```python
from build123d import *

# Parameters (mm, degrees)
F3_DEPTH      = 1400
F4_R          = 12
F4_R_2        = 8
F5_DEPTH      = 3
F5_DEPTH_BACK = 43
F6_DEPTH      = 63
F4_R_3        = 2
F7_DEPTH      = 50000


with BuildPart() as f3:
    # F2 (on Right) → F3 (new body)
    with BuildSketch(Plane.YZ):
        with BuildLine():
            Line((18.886194054, 20.0493852866), (-17.113805946, 20.0493852866))
            ThreePointArc((-17.113805946, 20.0493852866), (-18.5280195083, 19.463598849), (-19.113805946, 18.0493852866))
            Line((-19.113805946, 18.0493852866), (-19.113805946, -17.9506147134))
            ThreePointArc((-19.113805946, -17.9506147134), (-18.5280195083, -19.3648282758), (-17.113805946, -19.9506147134))
            Line((-17.113805946, -19.9506147134), (18.886194054, -19.9506147134))
            ThreePointArc((18.886194054, -19.9506147134), (20.3004076164, -19.3648282758), (20.886194054, -17.9506147134))
            Line((20.886194054, -17.9506147134), (20.886194054, 18.0493852866))
            ThreePointArc((20.886194054, 18.0493852866), (20.3004076164, 19.463598849), (18.886194054, 20.0493852866))
        make_face()
        with BuildLine():
            Line((-16.113805946, -14.9506147134), (-16.113805946, 15.0493852866))
            ThreePointArc((-16.113805946, 15.0493852866), (-15.5280195083, 16.463598849), (-14.113805946, 17.0493852866))
            Line((-14.113805946, 17.0493852866), (17.886194054, 17.0493852866))
            Line((17.886194054, 17.0493852866), (17.886194054, -14.9506147134))
            ThreePointArc((17.886194054, -14.9506147134), (17.3004076164, -16.3648282758), (15.886194054, -16.9506147134))
            Line((15.886194054, -16.9506147134), (-14.113805946, -16.9506147134))
            ThreePointArc((-14.113805946, -16.9506147134), (-15.5280195083, -16.3648282758), (-16.113805946, -14.9506147134))
        make_face(mode=Mode.SUBTRACT)
    extrude(amount=-F3_DEPTH)

    # F4 (on face) → F5 (join, two sides)
    with BuildSketch(Plane.XZ.offset(19.113805946)) as f5_sk:
        with Locations((-780, 0.0493852866)):
            Circle(F4_R)
        with Locations((-780, 0.0493852866)):
            Circle(F4_R_2, mode=Mode.SUBTRACT)
    extrude(amount=F5_DEPTH)
    extrude(f5_sk.sketch, amount=-F5_DEPTH_BACK)

    # F6 (cut): a face of the model
    f6_faces = [f3.faces().sort_by_distance(p)[0] for p in [
        (-780, 20.886194054, 0.0493852866),
    ]]
    extrude(f6_faces, amount=-F6_DEPTH, mode=Mode.SUBTRACT)

    # F4 (on face) → F7 (cut)
    with BuildSketch(Plane.XZ.offset(19.113805946)):
        with Locations((-44, 0)):
            Circle(F4_R_3)
        with Locations((-12, 0)):
            Circle(F4_R_3)
    extrude(amount=-F7_DEPTH, mode=Mode.SUBTRACT)


solid = f3.part
```
Read the model definition and answer for the solid it produces. Units are mm, in the model's axes. A direction names the side the tool comes from. Give positions to 0.01 mm unless a question says otherwise; leave off trailing zeros. Order: outer loops, then holes, each group sorted by start corner. A loop starts at its lowest first (then second) coordinate and runs counter-clockwise, first axis right, second up. Notation, with made-up numbers: (26, 13) -> (75, 13) arc R25 ccw to (75, 44) -> close; hole circle Ø4 at (1, -34.75). An arc over 180 degrees is marked (long way). One line per item, written item: value. Start each with the question number.
(1) The part is cut by section A-A (x = -241.5). Determine the outline of the cut face in (y, z), and give its area (3 significant figures).
(2) A tool of negligible diameter and unlimited length cuts with its end or side. For faces 1 (the flat face through (-690, 1, -16.951)), 2 (the flat face through (-778, 23.886, -8)), 3 (the cylindrical face through (-768.554, -20.593, 3.654)), 4 (the flat face through (0, 18.4, 0.3)), 5 (the flat face through (-690, 17.886, 1)), from which of +Z, -Z, +X, -X, +Y, -Y can it reach the whole face along a straight path? Write none if from no direction.
(3) Flat-ended cylindrical pins translate along their axes: P1, Ø4.5, axis at x = -44, z = 0, coming from the -Y side; P2, Ø14.5, axis at x = -780, z = 0.05, coming from the -Y side; P3, Ø5, axis at x = -1196.5, z = -11.5, coming from the +Y side; P4, Ø2, axis at y = -11, z = 10.5, coming from the +X side (3 decimals). Find the tip coordinate at first contact, or state that the pin passes through.
(4) Straight lines are drawn through the part: L1, parallel to X at y = 9, z = -1; L2, parallel to X at y = 4.5, z = 2; L3, parallel to Y at x = -1132.5, z = 1. For each, find the intervals that lie inside material, in ascending order.
(5) The part is cut by section B-B (y = -1). Determine the outline of the cut face in (x, z).
(6) For a pull along Z with two mould halves and no side action, classify faces 6 (the cylindrical face through (-768.554, 0.648, 3.654)), 7 (the cylindrical face through (-768.554, 22.365, 3.654)), 8 (the flat face through (-690, 1, 20.049)) as released by +Z, released by -Z, zero draft, split by the parting line, or undercut.
Taken from the geometry:
1. outline: (-19.11, -17.95) arc R2 ccw to (-17.11, -19.95) -> (18.89, -19.95) arc R2 ccw to (20.89, -17.95) -> (20.89, 18.05) arc R2 ccw to (18.89, 20.05) -> (-17.11, 20.05) arc R2 ccw to (-19.11, 18.05) -> close; hole (-16.11, -14.95) arc R2 ccw to (-14.11, -16.95) -> (15.89, -16.95) arc R2 ccw to (17.89, -14.95) -> (17.89, 17.05) -> (-14.11, 17.05) arc R2 ccw to (-16.11, 15.05) -> close
1. area: 443 mm^2
2. face 1: +X, -X
2. face 2: +Z, -Z, +X, -X, +Y
2. face 3: -Y
2. face 4: +Z, -Z, +X, +Y, -Y
2. face 5: none
3. P1: y = -19.11
3. P2: through
3. P3: y = 20.89
3. P4: x = -772.605
4. L1: -791.95 to -787.93, -772.07 to -768.05
4. L2: -791.84 to -787.76, -772.24 to -768.16
4. L3: -19.11 to -16.11, 17.89 to 20.89
5. outline: (-1400, -19.95) -> (0, -19.95) -> (0, -16.95) -> (-1400, -16.95) -> close; (-1400, 17.05) -> (0, 17.05) -> (0, 20.05) -> (-1400, 20.05) -> close; circle Ø24 at (-780, 0.05); hole circle Ø16 at (-780, 0.05)
6. face 6: undercut
6. face 7: split by the parting line
6. face 8: released by +Z
